```python
from build123d import *

# Parameters (mm, degrees)
SKETCH_1_R          = 5
EXTRUDE_1_DEPTH     = 532
SKETCH_2_W          = 3.43195358
SKETCH_2_H          = 1
SKETCH_2_W_2        = 4.632623125
CHAMFER_1_SIZE      = 0.5
SKETCH_3_W          = 38.697285924
SKETCH_3_H          = 59.202017993
CUT_EXTRUDE_1_DEPTH = 10
CHAMFER_2_SIZE      = 0.5


with BuildPart() as part:
    # 草图1 → 拉伸1 (new body)
    with BuildSketch(Plane.XY):
        Circle(SKETCH_1_R)
    extrude(amount=EXTRUDE_1_DEPTH)

    # 草图2 → 切除-旋转2 (revolve, cut)
    with BuildSketch(Plane(origin=(0, 0, 0), x_dir=(1, 0, 0), z_dir=(0, 1, 0)), mode=Mode.PRIVATE) as cut_revolve_2_sk:
        with Locations((-6.36597679, -469)):
            Rectangle(SKETCH_2_W, SKETCH_2_H)
        with Locations((-6.966311563, -63)):
            Rectangle(SKETCH_2_W_2, SKETCH_2_H)
    revolve(cut_revolve_2_sk.sketch.rotate(Axis((0, 0, 532), (0, 0, -1)), 180), axis=Axis((0, 0, 532), (0, 0, -1)), mode=Mode.SUBTRACT)

    # 倒角1
    chamfer_1_edges = [part.edges().sort_by_distance(p)[0] for p in [
        (-5, 0, 0),
        (-5, 0, 532),
    ]]
    chamfer(chamfer_1_edges, length=CHAMFER_1_SIZE)

    # 草图3 → 切除-拉伸1 (cut, symmetric)
    with BuildSketch(Plane(origin=(0, 0, 0), x_dir=(1, 0, 0), z_dir=(0, 1, 0))):
        with Locations((7.437997044, -520.101008997)):
            Rectangle(SKETCH_3_W, SKETCH_3_H)
    extrude(amount=CUT_EXTRUDE_1_DEPTH, both=True, mode=Mode.SUBTRACT)

    # 倒角2
    chamfer_2_edges = [part.edges().sort_by_distance(p)[0] for p in [
        (-5, 0, 490.5),
    ]]
    chamfer(chamfer_2_edges, length=CHAMFER_2_SIZE)


solid = part.part
```
Could you check a few things on this model? Use its own coordinates, in mm. A direction names the side the tool comes from. Give positions to 0.01 mm unless a question says otherwise; leave off trailing zeros. Loops run counter-clockwise (first coordinate to the right, second up) from the corner with the lowest first, then second, coordinate; pieces in that order, holes last. Notation, with made-up numbers: (20.5, 27) - (56.5, 27) arc R16 cw to (56.5, 47) - close; hole circle Ø1 at (27, -8.5). An arc over 180 degrees is marked (long way). Answer in a Markdown table with one row per item. Add a question column.
Q1. Which directions (+Z, -Z, +X, -X, +Y, -Y) give clear straight access to the entire face, cutting with the end or side of a thin tool? Please do faces 1 (the face through (-1.08, -4.88, 263.16)), 2 (the face through (4.295, 1.781, 62.993)).
Q2. For pin 1 (4 mm diameter, centred on x = -2, y = -3.5, fed in from -Z); pin 2 (1 mm diameter, centred on x = 2, z = 160.5, fed in from +Y); pin 3 (1.5 mm diameter, centred on x = -3, z = 399, fed in from -Y), each with a flat end and sliding along its axis, tell me the tip position at first contact or that it passes through.
Q3. We'd pull the mould along Z, two halves only. Please class faces 3 (the face through (2.5, -3.92, 468.99)), 4 (the face through (0, 0, 490.5)), 5 (the face through (0, 0, 0)): +Z half, -Z half, draft (parallel to the pull), parting line (faces both ways), or undercut.
Q4. If we section it at A-A (z = 355): List the corners of the cut face in (x, y) for me.
Q5. Please list where these lines run through material, in increasing order: L1, parallel to Z at x = 3.75, y = 3.25; L2, parallel to Z at x = -4.5, y = -1.75; L3, parallel to Y at x = -0.5, z = 345. Write a range as from..to.
The answers:
| question | item | result |
|---|---|---|
| 1 | face 1 | +Z, -Z |
| 1 | face 2 | none |
| 2 | pin 1 | stops at z = 0 |
| 2 | pin 2 | stops at y = 4.77 |
| 2 | pin 3 | stops at y = -4.47 |
| 3 | face 3 | undercut |
| 3 | face 4 | +Z half |
| 3 | face 5 | -Z half |
| 4 | outline | circle Ø10 at (0, 0) |
| 5 | L1 | z = 0.46..62.5, 63.5..468.5, 469.5..490.04 |
| 5 | L2 | z = 0.33..62.5, 63.5..468.5, 469.5..490.17 |
| 5 | L3 | y = -4.97..4.97 |
